Source: three-view drawing plus pictorial views. Frame: mm from the lowest corner of the part. A direction names the side the tool comes from. Round coordinates to 2 decimals unless told otherwise and drop trailing zeros. Order: outer loops, then holes, each group sorted by start corner. A loop starts at its lowest first (then second) coordinate and runs counter-clockwise, first axis right, second up. Notation, with made-up numbers: (49.5, 38) - (53.5, 38) arc R14 ccw to (53.5, 52) - close; hole circle Ø1 at (-15, 54.25). An arc over 180 degrees is marked (long way). One line per item, written item: value. Start each with the question number.
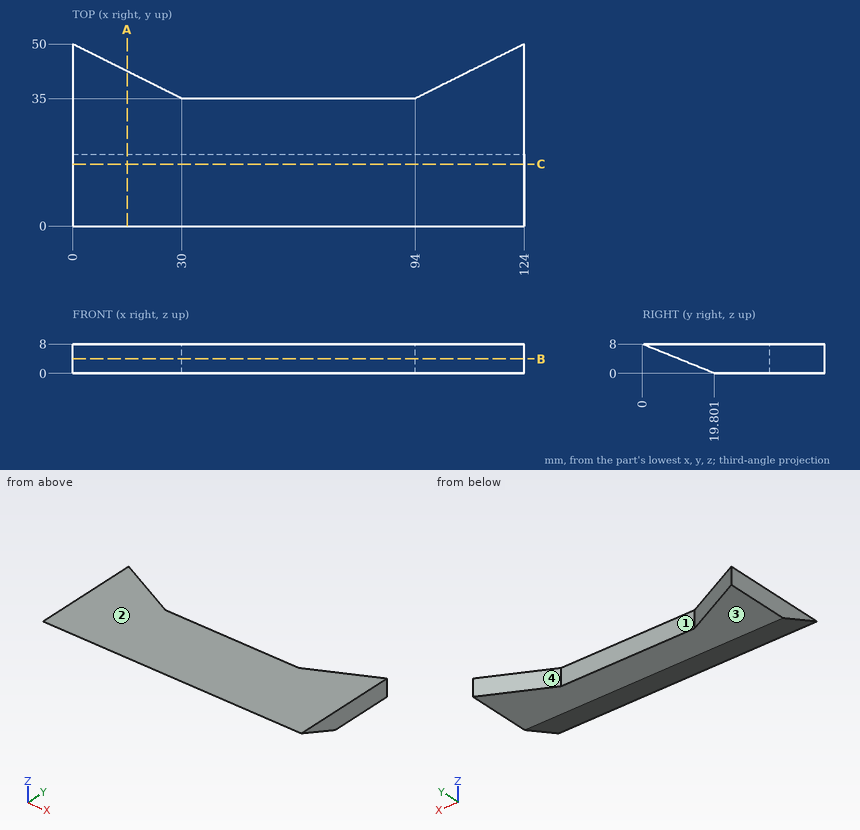
Item 1: First-contact query: pin 1 Ø1.5 at (x, y) = (78, 16.5) entering from -Z; pin 2 Ø6 at (x, y) = (67.5, 8.5) entering from -Z; pin 3 Ø1.5 at (x, z) = (60, 5) entering from -Y. Flat tips, straight axial feed; report the tip coordinate or a pass-through.
Item 2: Section query B-B on z = 4. Return loops of the section in (x, y).
Item 3: Section query C-C on y = 17. Return loops of the section in (x, z), and give its area (3 significant figures).
Item 4: Line query: L1, parallel to X at y = 37, z = 5.5; L2, parallel to X at y = 39, z = 2; L3, parallel to Z at x = 39.5, y = 6.5. Output: solid intervals per line, ascending.
Item 5: Pull-direction query (X, two-part tool) for the marked faces 1 and 2; classes: released by +X, released by -X, zero draft, split by the parting line, or undercut.
Item 6: Reachability of the marked faces 3 and 4 from +Z, -Z, +X, -X, +Y, -Y: full face, straight path, thin tool, end or side. Return the list, or none.
Item 7: Section query A-A on x = 15. Return loops of the section in (y, z), and give its area (3 significant figures).
Geometry results:
1. pin 1: stops at z = 1.03
1. pin 2: stops at z = 3.35
1. pin 3: stops at y = 5.57
2. outline: (0, 9.9) - (124, 9.9) - (124, 50) - (94, 35) - (30, 35) - (0, 50) - close
3. outline: (0, 1.13) - (124, 1.13) - (124, 8) - (0, 8) - close
3. area: 852 mm^2
4. L1: x = 0 to 26, 98 to 124
4. L2: x = 0 to 22, 102 to 124
4. L3: z = 5.37 to 8
5. face 1: undercut
5. face 2: zero draft
6. face 3: -Z, +X, -X, +Y, -Y
6. face 4: +Z, -Z, +Y
7. outline: (0, 8) - (19.8, 0) - (42.5, 0) - (42.5, 8) - close
7. area: 261 mm^2
